from build123d import *

# Parameters (mm, degrees)
F0_W      = 50
F0_H      = 50
F0_R      = 1.5
F1_DEPTH  = 1.6
F2_W      = 12.2
F2_H      = 50
F3_DEPTH  = 7.77
F4_R      = 5.1
F5_DEPTH  = 11.5
F6_W      = 9.7
F6_H      = 9.7
F7_DEPTH  = 11.1
F8_R      = 3.45
F9_DEPTH  = 5
F10_R     = 3
F11_DEPTH = 1.5
F13_DEPTH = 8.5


with BuildPart() as f1:
    # F0 (on Top) → F1 (new body)
    with BuildSketch(Plane.XY):
        Rectangle(F0_W, F0_H)
        with Locations((-6.5, -21.5)):
            Circle(F0_R, mode=Mode.SUBTRACT)
        with Locations((21.5, -21.5)):
            Circle(F0_R, mode=Mode.SUBTRACT)
        with Locations((21.5, 21.5)):
            Circle(F0_R, mode=Mode.SUBTRACT)
    extrude(amount=F1_DEPTH)

    # F2 (on face) → F3 (join)
    with BuildSketch(Plane.XY.offset(1.6)):
        with Locations((8.2, 0)):
            Rectangle(F2_W, F2_H)
    extrude(amount=F3_DEPTH)

    # F4 (on face) → F5 (join)
    with BuildSketch(Plane.XY.offset(1.6)):
        with Locations((-18, 15.1)):
            Circle(F4_R)
        with Locations((-5, 15.1)):
            Circle(F4_R)
    extrude(amount=F5_DEPTH)

    # F6 (on face) → F7 (join)
    with BuildSketch(Plane.XY.offset(1.6)):
        with Locations((-22.15, -17.35)):
            Rectangle(F6_W, F6_H)
    extrude(amount=F7_DEPTH)

    # F8 (on face) → F9 (join)
    with BuildSketch(Plane(origin=(-27, 0, 0), x_dir=(0, -1, 0), z_dir=(-1, 0, 0))):
        with Locations((17.35, 7.7)):
            Circle(F8_R)
    extrude(amount=F9_DEPTH)

    # F10 (on face) → F11 (join)
    with BuildSketch(Plane(origin=(-32, 0, 0), x_dir=(0, -1, 0), z_dir=(-1, 0, 0))):
        with Locations((17.35, 7.7)):
            Circle(F10_R)
    extrude(amount=F11_DEPTH)

    # F12 (on face) → F13 (join)
    with BuildSketch(Plane(origin=(-33.5, 0, 0), x_dir=(0, -1, 0), z_dir=(-1, 0, 0))):
        Polygon((16.880697, 4.736935), (16.880697, 10.663065), (16.577458, 10.077641), (15.988029, 10.37302), (15.880537, 9.722542), (15.22868, 9.82132), (15.327458, 9.169463), (14.67698, 9.061971), (14.972359, 8.472542), (14.386935, 8.169303), (14.85, 7.7), (14.386935, 7.230697), (14.972359, 6.927458), (14.67698, 6.338029), (15.327458, 6.230537), (15.22868, 5.57868), (15.880537, 5.677458), (15.988029, 5.02698), (16.577458, 5.322359), align=None)
        Polygon((18.122542, 10.077641), (17.819303, 10.663065), (17.819303, 4.736935), (18.122542, 5.322359), (18.711971, 5.02698), (18.819463, 5.677458), (19.47132, 5.57868), (19.372542, 6.230537), (20.02302, 6.338029), (19.727641, 6.927458), (20.313065, 7.230697), (19.85, 7.7), (20.313065, 8.169303), (19.727641, 8.472542), (20.02302, 9.061971), (19.372542, 9.169463), (19.47132, 9.82132), (18.819463, 9.722542), (18.711971, 10.37302), align=None)
    extrude(amount=F13_DEPTH)


solid = f1.part
Check sheet for the modelled part. Datum: model origin and axes. Units: mm. A direction names the side the tool comes from. Round coordinates to 2 decimals unless told otherwise and drop trailing zeros. Loops run counter-clockwise (first coordinate to the right, second up) from the corner with the lowest first, then second, coordinate; pieces in that order, holes last. Notation, with made-up numbers: (25.25, -7) - (45.25, -7) arc R17 cw to (45.25, 25) - close; hole circle Ø10 at (63.25, 39). An arc over 180 degrees is marked (long way). Answer as CSV lines item,"result". Start each with the question number.
Item 1: Section check D-D (y = -4). Record the boundary of the cut face in (x, z), and give its area (3 significant figures).
Item 2: Depth check by flat-ended pin: P1, Ø5, axis at y = -18.5, z = 7.5, coming from the +X side; P2, Ø5, axis at x = -31, z = 9.5, coming from the -Y side; P3, Ø2, axis at x = 7.5, y = 8, coming from the +Z side; P4, Ø2.5, axis at x = 21.5, y = -21.5, coming from the +Z side. Enter the tip coordinate at first touch or a pass-through.
Item 3: Section check A-A (z = 3.5). Record the boundary of the cut face in (x, y), and give its area (3 significant figures).
Item 4: Section check B-B (x = 21.5). Record the boundary of the cut face in (y, z), and give its area (3 significant figures).
Item 5: Scan lines: line 1 (Y direction, x = 21.5, z = 1.15); line 2 (Z direction, x = 3, y = -22); line 3 (Z direction, x = -1.5, y = -16). Record each from-to range of solid material in increasing order. Write a range as [from, to].
Item 6: Section check C-C (x = -6.5). Record the boundary of the cut face in (y, z).
Item 7: Set-up check for faces 4 (the flat face through (8, 0, 9.37)), 5 (the cylindrical face through (-29.46, -20.64, 8.74)), 6 (the flat face through (-22, -12.5, 7)), 7 (the cylindrical face through (-15.26, 19.4, 7.27)): record each of +Z, -Z, +X, -X, +Y, -Y from which the full face is reachable in a straight line by a thin tool's end or side.
Item 8: Release check for a two-part mould opening along Y. For faces 1 (the flat face through (-18, 15, 13.1)), 2 (the flat face through (-12, 0, 1.6)), 3 (the cylindrical face through (-8.8, 18.5, 7.3)) record: +Y half, -Y half, draft (parallel to the pull), parting line (faces both ways), or undercut.
Report:
1,outline,"(-25, 0) - (25, 0) - (25, 1.6) - (14.3, 1.6) - (14.3, 9.37) - (2.1, 9.37) - (2.1, 1.6) - (-25, 1.6) - close"
1,area,"175 mm2"
2,P1,"stops at x = 14.3"
2,P2,"stops at y = -20.8"
2,P3,"stops at z = 9.37"
2,P4,"passes through"
3,outline,"(-27, -22.2) - (-17.3, -22.2) - (-17.3, -12.5) - (-27, -12.5) - close; circle Ø10.2 at (-18, 15.1); circle Ø10.2 at (-5, 15.1); (2.1, -25) - (14.3, -25) - (14.3, 25) - (2.1, 25) - close"
3,area,"868 mm2"
4,outline,"(-25, 0) - (-23, 0) - (-23, 1.6) - (-25, 1.6) - close; (-20, 0) - (20, 0) - (20, 1.6) - (-20, 1.6) - close; (23, 0) - (25, 0) - (25, 1.6) - (23, 1.6) - close"
4,area,"70.4 mm2"
5,line 1,"y = [-25, -23], [-20, 20], [23, 25]"
5,line 2,"z = [0, 9.37]"
5,line 3,"z = [0, 1.6]"
6,outline,"(-25, 0) - (-23, 0) - (-23, 1.6) - (-25, 1.6) - close; (-20, 0) - (25, 0) - (25, 1.6) - (19.97, 1.6) - (19.97, 13.1) - (10.23, 13.1) - (10.23, 1.6) - (-20, 1.6) - close"
7,face 4,"+Z, +X, +Y, -Y"
7,face 5,"-X"
7,face 6,"+Z, -X"
7,face 7,"+Z"
8,face 1,"draft"
8,face 2,"undercut"
8,face 3,"parting line"
